Read the model definition and answer for the solid it produces. Units are mm, in the model's axes. Coordinates: 2 decimals unless noted, no trailing zeros. Write each loop counter-clockwise with the first axis right and the second up, starting at its lowest first coordinate (ties: lowest second). Pieces come first, ordered by that corner, then holes. Notation, with made-up numbers: (19, -4.75) -> (41, -4.75) arc R31 ccw to (41, 30.25) -> close; hole circle Ø9 at (85.5, 54.25). An arc over 180 degrees is marked (long way). One line per item, written item: value. Start each with the question number.
1. Find section B-B, the plane z = -58. Write down the section's boundary in (x, y), and give its area (3 significant figures).
2. Given P1, Ø0.8, axis at x = 0, y = -26, coming from the +Z side; P2, Ø0.8, axis at x = 0, y = -26.5, coming from the -Z side; P3, Ø0.8, axis at x = 0.5, z = -16.5, coming from the -Y side, each flat-ended and moving along its own axis, determine where each tip first touches the part or whether it passes through.
3. Consider line 1 along Z through (x, y) = (-0.15, 23); line 2 along Y through (x, z) = (0.45, -52). Determine where each line is inside the solid, lowest interval first.
4. Find section A-A, the plane y = -19. Write down the section's boundary in (x, z), and give its area (4 significant figures).
```python
from build123d import *

# Parameters (mm, degrees)
BOSS_EXTRUDE1_DEPTH = 1.25


with BuildPart() as part:
    # Sketch1 → Boss-Extrude1 (new, symmetric)
    with BuildSketch(Plane(origin=(0, 0, 0), x_dir=(0, 0, -1), z_dir=(1, 0, 0))):
        Polygon((10, -27.5), (-10, -27.5), (-10, -25), (-26.666666667, -25), (-26.666666667, -27.5), (-46.666666667, -27.5), (-46.666666667, -25), (-63.333333333, -25), (-63.333333333, -27.5), (-83.333333333, -27.5), (-83.333333333, -25), (-95.5, -25), (-95.5, -10), (-98, -10), (-98, 10), (-95.5, 10), (-95.5, 25), (-83.333333333, 25), (-83.333333333, 27.5), (-63.333333333, 27.5), (-63.333333333, 25), (-46.666666667, 25), (-46.666666667, 27.5), (-26.666666667, 27.5), (-26.666666667, 25), (-10, 25), (-10, 27.5), (10, 27.5), (10, 25), (26.666666667, 25), (26.666666667, 27.5), (46.666666667, 27.5), (46.666666667, 25), (63.333333333, 25), (63.333333333, 27.5), (83.333333333, 27.5), (83.333333333, 25), (95.5, 25), (95.5, 10), (98, 10), (98, -10), (95.5, -10), (95.5, -25), (83.333333333, -25), (83.333333333, -27.5), (63.333333333, -27.5), (63.333333333, -25), (46.666666667, -25), (46.666666667, -27.5), (26.666666667, -27.5), (26.666666667, -25), (10, -25), align=None)
    extrude(amount=BOSS_EXTRUDE1_DEPTH, both=True)


solid = part.part
```
Answer block:
1. outline: (-1.25, -25) -> (1.25, -25) -> (1.25, 25) -> (-1.25, 25) -> close
1. area: 125 mm2
2. P1: stops at z = 83.33
2. P2: stops at z = -83.33
2. P3: stops at y = -25
3. line 1: z = -95.5 to 95.5
3. line 2: y = -25 to 25
4. outline: (-1.25, -95.5) -> (1.25, -95.5) -> (1.25, 95.5) -> (-1.25, 95.5) -> close
4. area: 477.5 mm2
